```python
from build123d import *

# Parameters (mm, degrees)
SKETCH2_R           = 4.7625
SKETCH2_R_2         = 3.175
BOSS_EXTRUDE1_DEPTH = 9.525
SKETCH3_R           = 6.35
SKETCH3_R_2         = 4.7625
BOSS_EXTRUDE2_DEPTH = 1.5875
SKETCH4_R           = 6.35
CUT_EXTRUDE1_DEPTH  = 3.175


with BuildPart() as part:
    # Sketch2 → Boss-Extrude1 (new body)
    with BuildSketch(Plane(origin=(0, 0, 0), x_dir=(1, 0, 0), z_dir=(0, 1, 0))):
        Circle(SKETCH2_R)
        Circle(SKETCH2_R_2, mode=Mode.SUBTRACT)
    extrude(amount=BOSS_EXTRUDE1_DEPTH)

    # Sketch3 → Boss-Extrude2 (add)
    with BuildSketch(Plane(origin=(0, 0, 0), x_dir=(1, 0, 0), z_dir=(0, 1, 0))):
        Circle(SKETCH3_R)
        Circle(SKETCH3_R_2, mode=Mode.SUBTRACT)
    extrude(amount=BOSS_EXTRUDE2_DEPTH)

    # Sketch4 → Cut-Extrude1 (cut)
    with BuildSketch(Plane(origin=(0, 9.525, 0), x_dir=(1, 0, 0), z_dir=(0, 1, 0))):
        Circle(SKETCH4_R)
    extrude(amount=-CUT_EXTRUDE1_DEPTH, mode=Mode.SUBTRACT)


solid = part.part
```
The listing builds one solid part. Answer for the finished solid, in the listing's coordinates (mm). Coordinates: 2 decimals unless noted, no trailing zeros. Loops run counter-clockwise (first coordinate to the right, second up) from the corner with the lowest first, then second, coordinate; pieces in that order, holes last. Notation, with made-up numbers: M 44,-37 L 100,-37 A11 ccw 100,-30 Z; hole C 16,68 d8. An arc over 180 degrees is marked long. Answer as a JSON object with one key per item and string values. Group by question number.
Item 1: Section D-D (x = 4.5) is taken. Write down the section's boundary in (y, z), and give its area (3 significant figures).
Item 2: Consider L1, parallel to Z at x = 0, y = 4.5 (1 decimal); L2, parallel to Z at x = 1.5, y = 4. Determine where each line is inside the solid, lowest interval first.
Item 3: Determine the mould class of faces 1 (the face through (-0.69, 3.13, 3.1)), 2 (the face through (-1.38, 0.78, 6.2)), 3 (the face through (-2, 0, -3)) for opening direction X: +X half, -X half, draft (parallel to the pull), parting line (faces both ways), or undercut.
Item 4: This flat-tipped pin is pushed along its axis until it touches: P1, Ø2, axis at y = 3.5, z = -5, coming from the +X side. Where does it stop, or does it pass through?
Solved:
{
 "1": {"outline": "M 0,-4.48 L 1.59,-4.48 L 1.59,-1.56 L 6.35,-1.56 L 6.35,1.56 L 1.59,1.56 L 1.59,4.48 L 0,4.48 Z", "area": "29.1 mm2"},
 "2": {"L1": "z = -4.8 to -3.2, 3.2 to 4.8", "L2": "z = -4.52 to -2.8, 2.8 to 4.52"},
 "3": {"face 1": "undercut", "face 2": "parting line", "face 3": "draft"},
 "4": {"P1": "stops at x = 2.58"}
}
